```python
from build123d import *

# Parameters (mm, degrees)
EXTRUDE_1_DEPTH          = 15
SKETCH_2_R               = 2.6
CUT_EXTRUDE_1_DEPTH      = 42.374516613
SKETCH_3_R               = 2.6
CUT_EXTRUDE_2_DEPTH      = 37.793554123
CUT_EXTRUDE_4_DEPTH      = 3.5
CUT_EXTRUDE_4_DEPTH_BACK = 14
SKETCH_5_R               = 4.25
CUT_EXTRUDE_5_DEPTH      = 3.5
CUT_EXTRUDE_5_DEPTH_BACK = 18
SKETCH_6_R               = 4.25


with BuildPart() as part:
    # 草图1 → 凸台-拉伸1 (new body)
    with BuildSketch(Plane(origin=(0, 0, 0), x_dir=(1, 0, 0), z_dir=(0, 1, 0))):
        Polygon((14.875, 5.775), (-15.125, -24.225), (-15.125, 5.775), align=None)
    extrude(amount=EXTRUDE_1_DEPTH)

    # 草图2 → 切除-拉伸1 (cut, through all)
    with BuildSketch(Plane.ZY.offset(15.125)):
        with Locations((12.225, 7.5)):
            Circle(SKETCH_2_R)
    extrude(amount=-CUT_EXTRUDE_1_DEPTH, mode=Mode.SUBTRACT)

    # 草图3 → 切除-拉伸2 (cut, through all)
    with BuildSketch(Plane(origin=(0, 0, -5.775), x_dir=(-1, 0, 0), z_dir=(0, 0, -1))):
        with Locations((-2.875, 7.5)):
            Circle(SKETCH_3_R)
    extrude(amount=-CUT_EXTRUDE_2_DEPTH, mode=Mode.SUBTRACT)

    # 草图5 → 切除-拉伸4 (cut, two sides: drawn at the far end of the back side and taken through both)
    with BuildSketch(Plane.ZY.offset(5.125).offset(-CUT_EXTRUDE_4_DEPTH_BACK)):
        with Locations(Location((12.225, 7.5, 0), (0, 0, 180))):
            Circle(SKETCH_5_R)
    extrude(amount=CUT_EXTRUDE_4_DEPTH + CUT_EXTRUDE_4_DEPTH_BACK, mode=Mode.SUBTRACT)

    # 草图6 → 切除-拉伸5 (cut, two sides: drawn at the far end of the back side and taken through both)
    with BuildSketch(Plane(origin=(0, 0, 4.225), x_dir=(-1, 0, 0), z_dir=(0, 0, -1)).offset(-CUT_EXTRUDE_5_DEPTH_BACK)):
        with Locations(Location((-2.875, 7.5, 0), (0, 0, 45.099127844))):
            Circle(SKETCH_6_R)
    extrude(amount=CUT_EXTRUDE_5_DEPTH + CUT_EXTRUDE_5_DEPTH_BACK, mode=Mode.SUBTRACT)


solid = part.part
```
The model under review builds one solid part; all positions refer to its coordinate system, in mm. A direction names the side the tool comes from. Round coordinates to 2 decimals unless told otherwise and drop trailing zeros. Loops run counter-clockwise (first coordinate to the right, second up) from the corner with the lowest first, then second, coordinate; pieces in that order, holes last. Notation, with made-up numbers: M 50,8.25 L 86,8.25 A26 cw 86,26.25 Z; hole C -25.75,30 d5. An arc over 180 degrees is marked long. Answer as a JSON object with one key per item and string values.
(1) Take a section at C-C on y = 1.5. Give the boundary of the cut face in (x, z) (3 decimals).
Resolved:
{"outline": "M -15.125,-5.775 L 14.875,-5.775 L -15.125,24.225 Z"}
(2) Clearance check with flat-ended pins moving along their axes: P1, Ø2, axis at y = 6, z = 21, coming from the +X side; P2, Ø5, axis at x = -8, y = 9, coming from the +Z side; P3, Ø8, axis at y = 6, z = 11, coming from the +X side. State where each tip first meets the part, or that it passes through.
Resolved:
{"P1": "x = -10.9", "P2": "z = 19.6", "P3": "x = 1.27"}
(3) Take a section at A-A on z = -1.75. Give the boundary of the cut face in (x, y) (3 decimals), and give its area (3 significant figures).
Resolved:
{"outline": "M -15.125,0 L 10.85,0 L 10.85,15 L -15.125,15 Z; hole C 2.875,7.5 d5.2", "area": "368 mm²"}
(4) To check wall thickness, follow line 1 along X through (y, z) = (5.5, -3.5) (3 decimals); line 2 along Z through (x, y) = (1, 4) (3 decimals); line 3 along Y through (x, z) = (-1, 5.5). State the ranges of each line that lie inside material, in increasing order.
Resolved:
{"line 1": "-15.125 to 1.214, 4.536 to 12.6", "line 2": "-5.775 to 0.725", "line 3": "0 to 5.75, 9.25 to 15"}
(5) Draft analysis for pull direction X (two halves, no side actions). For faces 4 (the cylindrical face through (3.439, 4.962, -2.57)), 5 (the flat face through (-15.125, 7, 9)), 6 (the cylindrical face through (-11.92, 5.92, 10.16)), state which applies: released by +X, released by -X, zero draft, split by the parting line, or undercut.
Resolved:
{"face 4": "undercut", "face 5": "released by -X", "face 6": "zero draft"}
(6) Take a section at D-D on z = 4.75. Give the boundary of the cut face in (x, y) (3 decimals), and give its area (3 significant figures).
Resolved:
{"outline": "M -15.125,0 L 4.35,0 L 4.35,3.514 A4.25 cw long 4.35,11.486 L 4.35,15 L -15.125,15 Z", "area": "251 mm²"}
(7) Take a section at B-B on y = 7.5. Give the boundary of the cut face in (x, z) (3 decimals), and give its area (3 significant figures).
Resolved:
{"outline": "M -15.125,-5.775 L 0.275,-5.775 L 0.275,0.725 L -1.375,0.725 L -1.375,7.975 L -8.625,7.975 L -8.625,9.625 L -15.125,9.625 Z; M -15.125,14.825 L -8.625,14.825 L -8.625,16.475 L -7.375,16.475 L -15.125,24.225 Z; M 5.475,-5.775 L 14.875,-5.775 L 7.125,1.975 L 7.125,0.725 L 5.475,0.725 Z", "area": "292 mm²"}
(8) Tool access review of faces 1 (the flat face through (-8.625, 10.3, 12.3)), 2 (the cylindrical face through (-1.18, 6.23, 4.09)), 3 (the flat face through (0, 7, -5.775)): name each direction out of +Z, -Z, +X, -X, +Y, -Y from which nothing blocks a thin tool from reaching the whole face with its end or side.
Resolved:
{"face 1": "+X", "face 2": "+Z", "face 3": "-Z, +X, -X, +Y, -Y"}
